```python
from build123d import *

# Parameters (mm, degrees)
SKETCH1_W           = 80
SKETCH1_H           = 80
BOSS_EXTRUDE1_DEPTH = 6
SKETCH2_R           = 11
SKETCH2_R_2         = 2.75
CUT_EXTRUDE1_DEPTH  = 7
SKETCH3_R           = 2.75
CUT_EXTRUDE2_DEPTH  = 7
CUT_EXTRUDE3_DEPTH  = 7


with BuildPart() as part:
    # Sketch1 → Boss-Extrude1 (new body)
    with BuildSketch(Plane(origin=(0, 0, 0), x_dir=(0, 0, -1), z_dir=(1, 0, 0))):
        with Locations((11.749387771, -15.012106538)):
            Rectangle(SKETCH1_W, SKETCH1_H)
    extrude(amount=BOSS_EXTRUDE1_DEPTH)

    # Sketch2 → Cut-Extrude1 (cut, through all)
    with BuildSketch(Plane(origin=(6, 0, 0), x_dir=(0, 0, -1), z_dir=(1, 0, 0))):
        with Locations((11.749387771, -25.911850923)):
            Circle(SKETCH2_R)
        with Locations((-18.250612229, 14.987893462)):
            Circle(SKETCH2_R_2)
        with Locations((41.749387771, 14.987893462)):
            Circle(SKETCH2_R_2)
        with Locations((11.749387771, 14.987893462)):
            Circle(SKETCH2_R_2)
    extrude(amount=-CUT_EXTRUDE1_DEPTH, mode=Mode.SUBTRACT)

    # Sketch3 → Cut-Extrude2 (cut, through all)
    with BuildSketch(Plane.ZY):
        with Locations((6.216594167, -7.956810044)):
            Circle(SKETCH3_R)
        with Locations((-11.741651274, -0.511852102)):
            Circle(SKETCH3_R)
        with Locations((-29.704428651, -7.945868985)):
            Circle(SKETCH3_R)
        with Locations((-37.149386593, -25.904114427)):
            Circle(SKETCH3_R)
        with Locations((-29.715369709, -43.866891803)):
            Circle(SKETCH3_R)
        with Locations((6.205653109, -43.877832862)):
            Circle(SKETCH3_R)
        with Locations((13.650611051, -25.91958742)):
            Circle(SKETCH3_R)
    extrude(amount=-CUT_EXTRUDE2_DEPTH, mode=Mode.SUBTRACT)

    # Sketch5 → Cut-Extrude3 (cut, through all)
    with BuildSketch(Plane(origin=(6, 0, 0), x_dir=(0, 0, -1), z_dir=(1, 0, 0))):
        with BuildLine():
            Line((-19.446404481, -5.087804094), (-28.250612229, 4.870195687))
            Line((-28.250612229, 4.870195687), (-37.780318954, -56.381008327))
            Line((-37.780318954, -56.381008327), (19.620213458, -79.7647401))
            Line((19.620213458, -79.7647401), (69.424766919, -54.649801307))
            Line((69.424766919, -54.649801307), (51.749387771, 4.870195687))
            Line((51.749387771, 4.870195687), (42.945180022, -5.087804094))
            ThreePointArc((42.945180022, -5.087804094), (11.749387771, -63.419428565), (-19.446404481, -5.087804094))
        make_face()
    extrude(amount=-CUT_EXTRUDE3_DEPTH, mode=Mode.SUBTRACT)


solid = part.part
```
Verification items for the finished model (mm, model axes). A direction names the side the tool comes from. Give positions to 0.01 mm unless a question says otherwise; leave off trailing zeros. Write each loop counter-clockwise with the first axis right and the second up, starting at its lowest first coordinate (ties: lowest second). Pieces come first, ordered by that corner, then holes. Notation, with made-up numbers: M -16,15 L 36,15 A21 ccw 36,36 Z; hole C 9,-1 d3. An arc over 180 degrees is marked long. One line per question, with ' | ' between items.
1) Section check A-A on y = -21.5. Enter the section's corners in (x, z).
Result:
outline: M 0,-49 L 6,-49 L 6,-21.83 L 0,-21.83 Z; M 0,-1.67 L 6,-1.67 L 6,25.5 L 0,25.5 Z
2) Gauge pin test, flat end, axial feed: pin 1 Ø12 at (y, z) = (-34.5, 3.5) entering from -X. Record the tip position at first contact, or that the pin passes through.
Result:
pin 1: stops at x = 0
3) Thickness scan on line 1 along Z through (x, y) = (2, -42); line 2 along Z through (x, y) = (1.5, -45); line 3 along Y through (x, z) = (1.25, -32). Record the ranges inside material, lowest first. Write a range as [from, to].
Result:
line 1: z = [-45.63, -31.73], [-27.7, 4.2], [8.21, 22.13] | line 2: z = [-44.04, -32.22], [-27.21, 3.7], [8.72, 20.54] | line 3: y = [-55.01, -45.4], [-42.34, -9.46], [-6.43, 24.99]
4) Set-up check for faces 4 (the flat face through (3.042, -0.179, 23.787)), 5 (the cylindrical face through (2.96, -7.12, -27.08)), 6 (the flat face through (3.04, -0.04, -47.41)): record each of +Z, -Z, +X, -X, +Y, -Y from which the full face is reachable in a straight line by a thin tool's end or side.
Result:
face 4: +Z, +X, -X | face 5: +X, -X | face 6: -Z, +X, -X
5) Section check B-B on z = 5. Enter the section's corners in (x, y).
Result:
outline: M 0,-55.01 L 6,-55.01 L 6,-46.35 L 0,-46.35 Z; M 0,-41.41 L 6,-41.41 L 6,-10.42 L 0,-10.42 Z; M 0,-5.49 L 6,-5.49 L 6,24.99 L 0,24.99 Z
6) Section check C-C on x = 1. State how many separate pieces and enclosed holes the cut face has, plus the area to 3 significant figures.
Result:
separate pieces: 1 | enclosed holes: 11 | area: 5,120 mm2
7) Mould release check, pull along Z, two halves, no side actions. Record for faces 1 (the flat face through (0, -14, -11)), 2 (the flat face through (3, 15, -51.749)), 3 (the cylindrical face through (2.958, -46.562, 5.61)): released by +Z, released by -Z, zero draft, split by the parting line, or undercut.
Result:
face 1: zero draft | face 2: released by -Z | face 3: undercut
